from build123d import *

# Parameters (mm, degrees)
F1_DEPTH = 190.5
F4_DEPTH = 73.025
F6_D     = 9.525
F7_D     = 9.525


with BuildPart() as f1:
    # F0 (on Top) → F1 (new body)
    with BuildSketch(Plane.XY):
        with BuildLine():
            Line((-7.9375, 3.373814), (0, 3.373814))
            Line((0, 3.373814), (0, 9.723814))
            Line((0, 9.723814), (-31.75, 9.723814))
            Line((-31.75, 9.723814), (-49.53, 9.723814))
            ThreePointArc((-49.53, 9.723814), (-50.428026, 9.35184), (-50.8, 8.453814))
            Line((-50.8, 8.453814), (-50.8, 4.643814))
            ThreePointArc((-50.8, 4.643814), (-50.428026, 3.745788), (-49.53, 3.373814))
            Line((-49.53, 3.373814), (-33.3375, 3.373814))
            Line((-33.3375, 3.373814), (-7.9375, 3.373814))
        make_face()
        with BuildLine():
            Line((0, 9.723814), (0, 3.373814))
            Line((0, 3.373814), (7.9375, 3.373814))
            Line((7.9375, 3.373814), (33.3375, 3.373814))
            Line((33.3375, 3.373814), (49.53, 3.373814))
            ThreePointArc((49.53, 3.373814), (50.428026, 3.745788), (50.8, 4.643814))
            Line((50.8, 4.643814), (50.8, 8.453814))
            ThreePointArc((50.8, 8.453814), (50.428026, 9.35184), (49.53, 9.723814))
            Line((49.53, 9.723814), (31.75, 9.723814))
            Line((31.75, 9.723814), (0, 9.723814))
        make_face()
        with BuildLine():
            Line((-31.75, 9.723814), (0, 9.723814))
            Line((0, 9.723814), (0, 22.423814))
            Line((0, 22.423814), (-29.21, 22.423814))
            ThreePointArc((-29.21, 22.423814), (-31.006051, 21.679865), (-31.75, 19.883814))
            Line((-31.75, 19.883814), (-31.75, 9.723814))
        make_face()
        with BuildLine():
            Line((0, 22.423814), (0, 9.723814))
            Line((0, 9.723814), (31.75, 9.723814))
            Line((31.75, 9.723814), (31.75, 19.883814))
            ThreePointArc((31.75, 19.883814), (31.006051, 21.679865), (29.21, 22.423814))
            Line((29.21, 22.423814), (0, 22.423814))
        make_face()
        with BuildLine():
            Line((-7.9375, 1.27), (-7.9375, 3.373814))
            Line((-7.9375, 3.373814), (-33.3375, 3.373814))
            Line((-33.3375, 3.373814), (-33.3375, 1.27))
            ThreePointArc((-33.3375, 1.27), (-32.965526, 0.371974), (-32.0675, 0))
            Line((-32.0675, 0), (-9.2075, 0))
            ThreePointArc((-9.2075, 0), (-8.309474, 0.371974), (-7.9375, 1.27))
        make_face()
        with BuildLine():
            Line((33.3375, 3.373814), (7.9375, 3.373814))
            Line((7.9375, 3.373814), (7.9375, 1.27))
            ThreePointArc((7.9375, 1.27), (8.309474, 0.371974), (9.2075, 0))
            Line((9.2075, 0), (32.0675, 0))
            ThreePointArc((32.0675, 0), (32.965526, 0.371974), (33.3375, 1.27))
            Line((33.3375, 1.27), (33.3375, 3.373814))
        make_face()
    extrude(amount=F1_DEPTH)

    # F3 (on offset) → F4 (join)
    with BuildSketch(Plane.XY.offset(95.25)):
        with BuildLine():
            Line((-21.843277, 58.076449), (-28.575, 22.225))
            Line((-28.575, 22.225), (0, 22.225))
            Line((0, 22.225), (0, 31.75))
            ThreePointArc((0, 31.75), (-17.104171, 39.783525), (-21.843277, 58.076449))
        make_face()
        with BuildLine():
            ThreePointArc((0, 76.2), (-14.191475, 71.079171), (-21.843277, 58.076449))
            ThreePointArc((-21.843277, 58.076449), (-17.104171, 39.783525), (0, 31.75))
            Line((0, 31.75), (0, 38.1))
            ThreePointArc((0, 38.1), (-15.875, 53.975), (0, 69.85))
            Line((0, 69.85), (0, 76.2))
        make_face()
        with BuildLine():
            Line((0, 31.75), (0, 22.225))
            Line((0, 22.225), (28.575, 22.225))
            Line((28.575, 22.225), (21.843277, 58.076449))
            ThreePointArc((21.843277, 58.076449), (17.104171, 39.783525), (0, 31.75))
        make_face()
        with BuildLine():
            ThreePointArc((21.843277, 58.076449), (14.191475, 71.079171), (0, 76.2))
            Line((0, 76.2), (0, 69.85))
            ThreePointArc((0, 69.85), (15.875, 53.975), (0, 38.1))
            Line((0, 38.1), (0, 31.75))
            ThreePointArc((0, 31.75), (17.104171, 39.783525), (21.843277, 58.076449))
        make_face()
    extrude(amount=F4_DEPTH)

    # F6 (through all)
    with Locations(Plane.XZ):
        with Locations((0, 180.975)):
            Hole(F6_D / 2)

    # F7 (through all)
    with Locations(Plane.XZ):
        with Locations((0, 9.525)):
            Hole(F7_D / 2)


solid = f1.part
Design review of the part built by this model. Coordinates are the model's own, in mm. A direction names the side the tool comes from. Coordinates: 2 decimals unless noted, no trailing zeros. Loops run counter-clockwise (first coordinate to the right, second up) from the corner with the lowest first, then second, coordinate; pieces in that order, holes last.
Item 1: Add section C-C (z = 44.5). Write out the cut boundary in (x, y), and give its area (3 significant figures).
Completed:
outline: (-50.8, 4.64) arc R1.27 ccw to (-49.53, 3.37) - (-33.34, 3.37) - (-33.34, 1.27) arc R1.27 ccw to (-32.07, 0) - (-9.21, 0) arc R1.27 ccw to (-7.94, 1.27) - (-7.94, 3.37) - (7.94, 3.37) - (7.94, 1.27) arc R1.27 ccw to (9.21, 0) - (32.07, 0) arc R1.27 ccw to (33.34, 1.27) - (33.34, 3.37) - (49.53, 3.37) arc R1.27 ccw to (50.8, 4.64) - (50.8, 8.45) arc R1.27 ccw to (49.53, 9.72) - (31.75, 9.72) - (31.75, 19.88) arc R2.54 ccw to (29.21, 22.42) - (-29.21, 22.42) arc R2.54 ccw to (-31.75, 19.88) - (-31.75, 9.72) - (-49.53, 9.72) arc R1.27 ccw to (-50.8, 8.45) - close
area: 1,620 mm2
Item 2: Clearance check with flat-ended pins moving along their axes: pin 1 (1.1 mm diameter, centred on y = 3, z = 55, fed in from -X); pin 2 (1.1 mm diameter, centred on y = 2.5, z = 120.5, fed in from +X); pin 3 (12.5 mm diameter, centred on x = 0, z = 9.525, fed in from -Y). State where each tip first meets the part, or that it passes through.
Completed:
pin 1: stops at x = -50.18
pin 2: stops at x = 33.34
pin 3: stops at y = 3.37
Item 3: Wall thickness on L1, parallel to Z at x = 0, y = 10; L2, parallel to Y at x = 7, z = 72.5; L3, parallel to Y at x = -27.5, z = 68: over which ranges is each line inside the solid? List them lowest first.
Completed:
L1: z = 0 to 4.76, 14.29 to 176.21, 185.74 to 190.5
L2: y = 3.37 to 22.42
L3: y = 0 to 22.42
Item 4: Add section B-B (x = 13). Write out the cut boundary in (y, z) (3 decimals), and give its area (3 significant figures).
Completed:
outline: (0, 0) - (22.424, 0) - (22.424, 95.25) - (44.864, 95.25) - (44.864, 168.275) - (22.424, 168.275) - (22.424, 190.5) - (0, 190.5) - close; (63.086, 95.25) - (72.001, 95.25) - (72.001, 168.275) - (63.086, 168.275) - close
area: 6,560 mm2
Item 5: For faces 1 (the flat face through (-41, 9.724, 94)), 2 (the flat face through (-42, 3.374, 94)), 3 (the flat face through (41, 3.374, 94)), 4 (the flat face through (0, 3.374, 94)), list the 3-axis set-ups (+Z, -Z, +X, -X, +Y, -Y) from which the entire face can be reached by the end or side of a thin tool; tool diameter is ignored.
Completed:
face 1: +Z, -Z, -X, +Y
face 2: +Z, -Z, -X, -Y
face 3: +Z, -Z, +X, -Y
face 4: +Z, -Z, -Y
Item 6: Add section D-D (y = 67). Write out the cut boundary in (x, z) (3 decimals), and give its area (3 significant figures).
Completed:
outline: (-18.008, 95.25) - (-9.076, 95.25) - (-9.076, 168.275) - (-18.008, 168.275) - close; (9.076, 95.25) - (18.008, 95.25) - (18.008, 168.275) - (9.076, 168.275) - close
area: 1,300 mm2
Item 7: Draft analysis for pull direction Z (two halves, no side actions). For faces 5 (the cylindrical face through (4.768, 69.117, 131.251)), 6 (the cylindrical face through (1.032, 13.032, 176.326)), 7 (the flat face through (-0.4, 37.7, 168.275)), state which applies: pulls with the +Z half, pulls with the -Z half, needs draft (parallel to the pull), parting line crosses it, or undercut.
Completed:
face 5: needs draft
face 6: undercut
face 7: pulls with the +Z half
